```python
from build123d import *

# Parameters (mm, degrees)
F1_DEPTH = 50.8
F2_W     = 12.071142
F2_H     = 88.9
F3_DEPTH = 50.8
F4_W     = 114.3
F4_H     = 50.605938
F5_DEPTH = 50.8


with BuildPart() as f1:
    # F0 (on Front) → F1 (new body)
    with BuildSketch(Plane.XZ):
        Polygon((61.682204, 59.341179), (-52.617796, 59.341179), (-52.617796, -29.558821), (-14.517796, -29.558821), (-14.517796, -16.858821), (23.582204, -16.858821), (23.582204, -29.558821), (61.682204, -29.558821), align=None)
    extrude(amount=F1_DEPTH)

    # F2 (on Right) → F3 (join)
    with BuildSketch(Plane.YZ):
        with Locations((6.035571, 14.272146)):
            Rectangle(F2_W, F2_H)
    extrude(amount=F3_DEPTH)

    # F4 (on Top) → F5 (join)
    with BuildSketch(Plane.XY):
        with Locations((5.460755, -25.302969)):
            Rectangle(F4_W, F4_H)
    extrude(amount=F5_DEPTH)


solid = f1.part
```
Design review of the part built by this model. Coordinates are the model's own, in mm. A direction names the side the tool comes from. Give positions to 0.01 mm unless a question says otherwise; leave off trailing zeros. Order: outer loops, then holes, each group sorted by start corner. A loop starts at its lowest first (then second) coordinate and runs counter-clockwise, first axis right, second up. Notation, with made-up numbers: (40, 35.25) -> (71, 35.25) arc R19 cw to (71, 51.25) -> close; hole circle Ø9 at (70.5, 31). An arc over 180 degrees is marked (long way). Write item = value, one per line. Start each with the question number.
(1) We need section B-B on y = -18. Write out the cut boundary in (x, z), plus the area to 3 significant figures.
(2) We need section C-C on z = 39.5. Write out the cut boundary in (x, y).
(3) For pin 1 (11.5 mm diameter, centred on x = 6, y = -13.5, fed in from -Z); pin 2 (14 mm diameter, centred on y = -27, z = -23.5, fed in from +X); pin 3 (1 mm diameter, centred on x = 62.5, y = -24, fed in from -Z), all flat-tipped, find the tip position at first contact; note any pin that passes through.
(4) Mouldability with a two-part tool opening along X and no side actions: class faces 1 (the face through (-34, -25, -29.559)), 2 (the face through (-14.518, -25, -23)), 3 (the face through (-52.618, -25, 16)) as +X half, -X half, draft (parallel to the pull), parting line (faces both ways), or undercut.
(5) We need section A-A on z = -21.5. Write out the cut boundary in (x, y).
(6) To check wall thickness, follow line 1 along X through (y, z) = (-30, -17); line 2 along X through (y, z) = (9, -6); line 3 along Y through (x, z) = (-37.5, 31.5). State the ranges of each line that lie inside material, in increasing order.
(7) For faces 4 (the face through (4, -25, -16.859)), 5 (the face through (50.8, 6, 15)), 6 (the face through (42, -25, -29.559)), list the 3-axis set-ups (+Z, -Z, +X, -X, +Y, -Y) from which the entire face can be reached by the end or side of a thin tool; tool diameter is ignored.
(8) We need section D-D on x = 10.5. Write out the cut boundary in (y, z), plus the area to 3 significant figures.
Numbers:
q1.outline = (-52.62, -29.56) -> (-14.52, -29.56) -> (-14.52, -16.86) -> (23.58, -16.86) -> (23.58, -29.56) -> (61.68, -29.56) -> (61.68, 0) -> (62.61, 0) -> (62.61, 50.8) -> (61.68, 50.8) -> (61.68, 59.34) -> (-52.62, 59.34) -> close
q1.area = 9,720 mm^2
q2.outline = (-52.62, -50.8) -> (61.68, -50.8) -> (61.68, -50.61) -> (62.61, -50.61) -> (62.61, 0) -> (50.8, 0) -> (50.8, 12.07) -> (0, 12.07) -> (0, 0) -> (-52.62, 0) -> close
q3.pin_1 = -16.86
q3.pin_2 = 61.68
q3.pin_3 = 0
q4.face_1 = draft
q4.face_2 = undercut
q4.face_3 = -X half
q5.outline = (-52.62, -50.8) -> (-14.52, -50.8) -> (-14.52, 0) -> (-52.62, 0) -> close; (0, 0) -> (23.58, 0) -> (23.58, -50.8) -> (61.68, -50.8) -> (61.68, 0) -> (50.8, 0) -> (50.8, 12.07) -> (0, 12.07) -> close
q6.line_1 = -52.62 to -14.52, 23.58 to 61.68
q6.line_2 = 0 to 50.8
q6.line_3 = -50.8 to 0
q7.face_4 = -Z, -Y
q7.face_5 = +Z, -Z, +X, +Y
q7.face_6 = -Z, +X, -X, -Y
q8.outline = (-50.8, -16.86) -> (0, -16.86) -> (0, -30.18) -> (12.07, -30.18) -> (12.07, 58.72) -> (0, 58.72) -> (0, 59.34) -> (-50.8, 59.34) -> close
q8.area = 4,940 mm^2
